from build123d import *

# Parameters (mm, degrees)
F1_DEPTH      = 50.8
F2_R          = 9.525
F3_DEPTH      = 50.801
F4_R          = 2.54
F5_W          = 63.5
F5_H          = 12.7
F6_DEPTH      = 39.6885
F6_DEPTH_BACK = 39.6885


with BuildPart() as f1:
    # F0 (on Top) → F1 (new body)
    with BuildSketch(Plane.XY):
        Polygon((-39.6875, 38.1), (-39.6875, -38.1), (39.6875, -38.1), (39.6875, 38.1), (15.875, 63.5), (15.875, 107.95), (-15.875, 107.95), (-15.875, 63.5), align=None)
    extrude(amount=F1_DEPTH)

    # F2 (on face) → F3 (cut, through all)
    with BuildSketch(Plane.XY.offset(50.8)):
        Circle(F2_R)
    extrude(amount=-F3_DEPTH, mode=Mode.SUBTRACT)

    # F4
    f4_edges = [f1.edges().sort_by_distance(p)[0] for p in [
        (-9.525, 0, 0),
        (-9.525, 0, 50.8),
        (9.525, 0, 25.4),
    ]]
    fillet(f4_edges, radius=F4_R)

    # F5 (on Right) → F6 (cut, two sides)
    with BuildSketch(Plane.YZ) as f6_sk:
        with Locations((0, 25.4)):
            Rectangle(F5_W, F5_H)
    extrude(amount=-F6_DEPTH, mode=Mode.SUBTRACT)
    extrude(f6_sk.sketch, amount=F6_DEPTH_BACK, mode=Mode.SUBTRACT)


solid = f1.part
Model file for the job. Use its own axes, mm. A direction names the side the tool comes from. Give positions to 0.01 mm unless a question says otherwise; leave off trailing zeros. Loops run counter-clockwise (first coordinate to the right, second up) from the corner with the lowest first, then second, coordinate; pieces in that order, holes last.
Item 1: Slice it at A-A (y = 0). Give the number of separate pieces and of enclosed holes in the cut face, plus the area to 3 significant figures.
Check values:
separate pieces: 4
enclosed holes: 0
area: 2,290 mm2
Item 2: Drill centre lines: line 1 along Z through (x, y) = (3, 21.5); line 2 along Y through (x, z) = (0, 44) (3 decimals); line 3 along Y through (x, z) = (33.5, 31.5). Where is each one in solid material? Low to high.
Check values:
line 1: z = 0 to 19.05, 31.75 to 50.8
line 2: y = -38.1 to -9.525, 9.525 to 107.95
line 3: y = -38.1 to -31.75, 31.75 to 44.7
Item 3: Slice it at D-D (x = -22). Write the cut outline in (y, z), plus the area to 3 significant figures.
Check values:
outline: (-38.1, 0) - (56.97, 0) - (56.97, 50.8) - (-38.1, 50.8) - close; hole (-31.75, 19.05) - (31.75, 19.05) - (31.75, 31.75) - (-31.75, 31.75) - close
area: 4,020 mm2
Item 4: Which spindle directions (+Z, -Z, +X, -X, +Y, -Y) get a long thin tool onto all of the face, cutting with end or side? Do faces 1 (the face through (15.875, 85, 25)), 2 (the face through (1, 31.75, 25)), 3 (the face through (-39.688, 1, 14)), 4 (the face through (-15.875, 86, 25)). Say none if no direction does.
Check values:
face 1: +Z, -Z, +X, +Y
face 2: +X, -X
face 3: +Z, -Z, -X, +Y, -Y
face 4: +Z, -Z, -X, +Y
Item 5: Drop flat-ended pins along their axis: P1, Ø1.5, axis at y = 93, z = 21, coming from the +X side (3 decimals); P2, Ø13.5, axis at y = 95.5, z = 35.5, coming from the -X side (3 decimals); P3, Ø10, axis at y = 57.5, z = 8, coming from the +X side. Give the stop position or say it passes through.
Check values:
P1: stops at x = 15.875
P2: stops at x = -15.875
P3: stops at x = 26.19
Item 6: Mould opens along Y. For faces 5 (the face through (39.688, -1, 14)), 6 (the face through (9, 7, 19.05)), 7 (the face through (-1, -38.1, 25)) say: +Y half, -Y half, draft (parallel to the pull), parting line (faces both ways), or undercut.
Check values:
face 5: draft
face 6: undercut
face 7: -Y half
Item 7: Slice it at B-B (x = 0). Write the cut outline in (y, z) (3 decimals).
Check values:
outline: (-38.1, 0) - (-12.065, 0) arc R2.54 ccw to (-9.525, 2.54) - (-9.525, 19.05) - (-31.75, 19.05) - (-31.75, 31.75) - (-9.525, 31.75) - (-9.525, 48.26) arc R2.54 ccw to (-12.065, 50.8) - (-38.1, 50.8) - close; (9.525, 2.54) arc R2.54 ccw to (12.065, 0) - (107.95, 0) - (107.95, 50.8) - (12.065, 50.8) arc R2.54 ccw to (9.525, 48.26) - (9.525, 31.75) - (31.75, 31.75) - (31.75, 19.05) - (9.525, 19.05) - close
